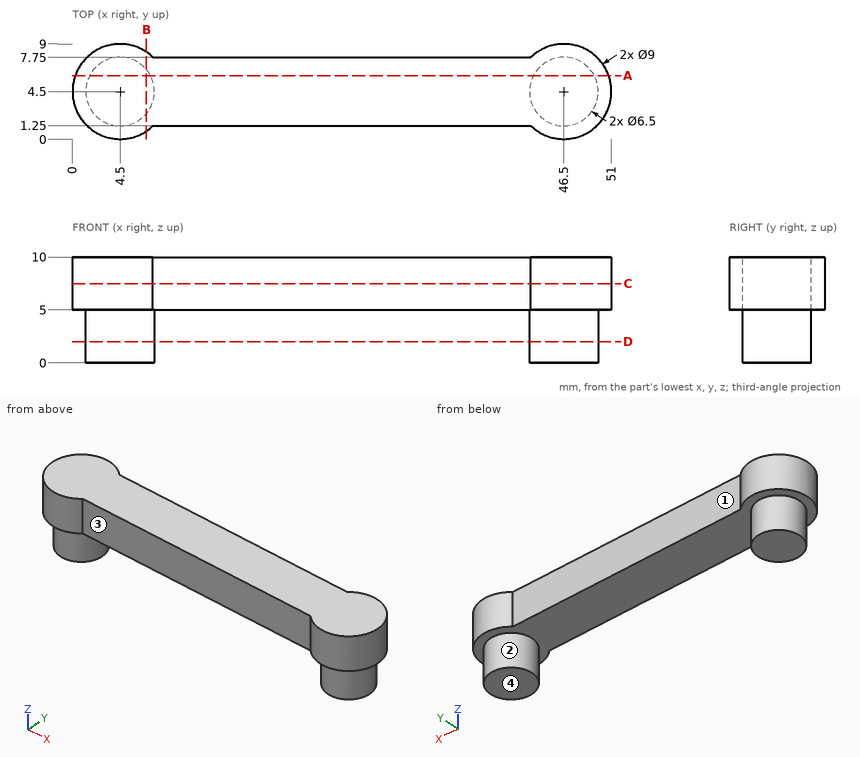
Answer from the drawing. Dimensions are ordinates in mm from the lowest x, y and z of the part. A direction names the side the tool comes from. Coordinates: 2 decimals unless noted, no trailing zeros. Loops run counter-clockwise (first coordinate to the right, second up) from the corner with the lowest first, then second, coordinate; pieces in that order, holes last. Notation, with made-up numbers: (4.25, -18) -> (27.25, -18) arc R9 cw to (27.25, -4) -> close; hole circle Ø7 at (36.5, 38.25). An arc over 180 degrees is marked (long way). Return JSON: item names as keys, results as strings.
Item 1: Find section C-C (z = 7.5). Determine the outline of the cut face in (x, y), plus the area to 3 significant figures.
Answers:
{"outline": "(7.61, 1.25) -> (43.39, 1.25) arc R4.5 ccw (long way) to (43.39, 7.75) -> (7.61, 7.75) arc R4.5 ccw (long way) to start", "area": "347 mm2"}
Item 2: Find section A-A (y = 6). Determine the outline of the cut face in (x, z).
Answers:
{"outline": "(0.26, 5) -> (1.62, 5) -> (1.62, 0) -> (7.38, 0) -> (7.38, 5) -> (43.62, 5) -> (43.62, 0) -> (49.38, 0) -> (49.38, 5) -> (50.74, 5) -> (50.74, 10) -> (0.26, 10) -> close"}
Item 3: Find section D-D (z = 2). Determine the outline of the cut face in (x, y).
Answers:
{"outline": "circle Ø6.5 at (4.5, 4.5); circle Ø6.5 at (46.5, 4.5)"}
Item 4: For the marked faces 1, 2, 3 and 4, determine the directions among +Z, -Z, +X, -X, +Y, -Y from which every point of the face is accessible in a straight line to the end or side of a thin tool.
Answers:
{"face 1": "+Z, -Z, +Y", "face 2": "-Z", "face 3": "+Z, -Z, -Y", "face 4": "-Z, +X, -X, +Y, -Y"}
Item 5: Flat-ended cylindrical pins translate along their axes: P1, Ø3, axis at x = 19.5, z = 3, coming from the -Y side; P2, Ø4, axis at x = 33.5, z = 8, coming from the +Y side; P3, Ø1, axis at x = 29.5, y = 5.5, coming from the -Z side; P4, Ø1, axis at y = 7, z = 8, coming from the -X side. Find the tip coordinate at first contact, or state that the pin passes through.
Answers:
{"P1": "passes through", "P2": "stops at y = 7.75", "P3": "stops at z = 5", "P4": "stops at x = 0.47"}
Item 6: Find the intervals of material crossed by probe 1 along Y at (x, z) = (14.5, 7.5); probe 2 along Z at (x, y) = (49.5, 7); probe 3 along X at (y, z) = (3.25, 3.25), in increasing order.
Answers:
{"probe 1": "y = 1.25 to 7.75", "probe 2": "z = 5 to 10", "probe 3": "x = 1.5 to 7.5, 43.5 to 49.5"}
Item 7: Find section B-B (x = 7). Determine the outline of the cut face in (y, z).
Answers:
{"outline": "(0.76, 5) -> (2.42, 5) -> (2.42, 0) -> (6.58, 0) -> (6.58, 5) -> (8.24, 5) -> (8.24, 10) -> (0.76, 10) -> close"}
